The listing builds one solid part. Answer for the finished solid, in the listing's coordinates (mm). A direction names the side the tool comes from. Coordinates: 2 decimals unless noted, no trailing zeros. Order: outer loops, then holes, each group sorted by start corner. A loop starts at its lowest first (then second) coordinate and runs counter-clockwise, first axis right, second up. Notation, with made-up numbers: (-4.75, -6) -> (17.25, -6) arc R22 cw to (17.25, 16) -> close; hole circle Ø3 at (14, 79). An arc over 180 degrees is marked (long way). Write each question's results on one line, items separated by ' | '. Start each with the question number.
(1) The part is cut by section C-C, the plane z = 3. Give the vertices of the cut face in (x, y) (3 decimals), then the cut area to 3 significant figures.
(2) The part is cut by section A-A, the plane y = 2.5. Give the vertices of the cut face in (x, z) (3 decimals), then the cut area to 3 significant figures.
(3) A tool of negligible diameter and unlimited length cuts with its end or side. For faces 5 (the face through (3.175, 0, 6)), 6 (the face through (-3.4, 0.2, 12.7)), from which of +Z, -Z, +X, -X, +Y, -Y can it reach the whole face along a straight path? Write none if from no direction.
(4) Straight lines are drawn through the part: L1, parallel to X at y = 1, z = 0.5 (3 decimals); L2, parallel to X at y = -6, z = 6; L3, parallel to Y at x = 0.5, z = 12.25. For each, find the intervals that lie inside material, in ascending order.
(5) Determine the mould class of faces 1 (the face through (0, 17.699, 6)), 2 (the face through (-14.303, 0, 6)), 3 (the face through (-3.175, 0, 6)), 4 (the face through (0.07, -6.35, 6.26)) for opening direction X: +X half, -X half, draft (parallel to the pull), parting line (faces both ways), or undercut.
(6) The part is cut by section B-B, the plane x = 0. Give the vertices of the cut face in (y, z), then the cut area to 3 significant figures.
```python
from build123d import *

# Parameters (mm, degrees)
F0_W     = 28.606172
F0_H     = 35.397082
F1_DEPTH = 12.7


with BuildPart() as f1:
    # F0 (on Top) → F1 (new body)
    with BuildSketch(Plane.XY):
        Rectangle(F0_W, F0_H)
        with BuildLine():
            Line((3.175, 3.175), (3.175, -3.175))
            ThreePointArc((3.175, -3.175), (0, -6.35), (-3.175, -3.175))
            Line((-3.175, -3.175), (-3.175, 3.175))
            ThreePointArc((-3.175, 3.175), (0, 6.35), (3.175, 3.175))
        make_face(mode=Mode.SUBTRACT)
    extrude(amount=F1_DEPTH)


solid = f1.part
```
Established:
1) outline: (-14.303, -17.699) -> (14.303, -17.699) -> (14.303, 17.699) -> (-14.303, 17.699) -> close; hole (-3.175, -3.175) arc R3.175 ccw to (3.175, -3.175) -> (3.175, 3.175) arc R3.175 ccw to (-3.175, 3.175) -> close | area: 941 mm^2
2) outline: (-14.303, 0) -> (-3.175, 0) -> (-3.175, 12.7) -> (-14.303, 12.7) -> close; (3.175, 0) -> (14.303, 0) -> (14.303, 12.7) -> (3.175, 12.7) -> close | area: 283 mm^2
3) face 5: +Z, -Z | face 6: +Z, +X, -X, +Y, -Y
4) L1: x = -14.303 to -3.175, 3.175 to 14.303 | L2: x = -14.3 to -1.45, 1.45 to 14.3 | L3: y = -17.7 to -6.31, 6.31 to 17.7
5) face 1: draft | face 2: -X half | face 3: undercut | face 4: undercut
6) outline: (-17.7, 0) -> (-6.35, 0) -> (-6.35, 12.7) -> (-17.7, 12.7) -> close; (6.35, 0) -> (17.7, 0) -> (17.7, 12.7) -> (6.35, 12.7) -> close | area: 288 mm^2
